Geometry check sheet. Reference: the model listing, model coordinates, mm. A direction names the side the tool comes from. Coordinates: 2 decimals unless noted, no trailing zeros. Loops run counter-clockwise (first coordinate to the right, second up) from the corner with the lowest first, then second, coordinate; pieces in that order, holes last. Notation, with made-up numbers: (-2.5, 11.25) - (48.5, 11.25) arc R29 ccw to (48.5, 46.25) - close; hole circle Ø6 at (81, 89.5). An arc over 180 degrees is marked (long way). Write each question's results on one line, items separated by ' | '. Start each with the question number.
(1) Sectioned sample at B-B (z = -4). Enter the section's corners in (x, y), plus the area to 3 significant figures.
(2) Material ranges on probe 1 along Z at (x, y) = (-8, -0.7); probe 2 along Y at (x, z) = (-9, -3.5); probe 3 along Z at (x, y) = (9, 24), recorded low to high.
(3) Sectioned sample at C-C (y = 19.5). Enter the section's corners in (x, z).
(4) Access from +Z, -Z, +X, -X, +Y, -Y to the whole of each face (thin tool, end or side, straight path). Record for faces 4 (the face through (-9.352, -0.74, 9.474)), 5 (the face through (-4, 0, -4)).
(5) Go/stop test with flat-tipped pins: pin 1 Ø1.8 at (x, y) = (8.5, 16.75) entering from -Z; pin 2 Ø12 at (x, y) = (-7.5, 7.5) entering from -Z; pin 3 Ø13 at (x, z) = (0, 0) entering from +Y. Record where each tip stops, or that it passes through.
(6) Sectioned sample at D-D (x = -8.5). Enter the section's corners in (y, z).
(7) Sectioned sample at A-A (z = 8). Enter the section's corners in (x, y).
(8) Mould release check, pull along X, two halves, no side actions. Record for faces 1 (the face through (-0.309, 33.497, 16.497)), 2 (the face through (9.352, -0.74, -9.474)), 3 (the face through (4, 14, 15.737)): pulls with the +X half, pulls with the -X half, needs draft (parallel to the pull), parting line crosses it, or undercut.
from build123d import *

# Parameters (mm, degrees)
SKETCH1_W                = 30
SKETCH1_H                = 30
SKETCH1_R                = 5
SKETCH1_R_2              = 2
BASE_FLANGE1_DEPTH       = 1.5
EDGE_FLANGE1_DEPTH       = 30
EDGE_FLANGE1_START       = -1.5
EDGE_FLANGE1_PROFILE_R   = 1.5
EDGE_FLANGE1_PROFILE_R_2 = 3.6
EDGE_FLANGE1_FLAT_DEPTH  = 1.5


# Sheet-metal steps are written as plain solids
with BuildPart() as part:
    # Sketch1 → Base-Flange1 (new body)
    with BuildSketch(Plane(origin=(0, 0, 0), x_dir=(1, 0, 0), z_dir=(0, 1, 0))):
        Rectangle(SKETCH1_W, SKETCH1_H)
        with Locations(Location((0, 0, 0), (0, 0, 270))):
            Circle(SKETCH1_R, mode=Mode.SUBTRACT)
        with Locations(Location((8, 8, 0), (0, 0, 270))):
            Circle(SKETCH1_R_2, mode=Mode.SUBTRACT)
        with Locations(Location((8, -8, 0), (0, 0, 270))):
            Circle(SKETCH1_R_2, mode=Mode.SUBTRACT)
        with Locations(Location((-8, -8, 0), (0, 0, 90))):
            Circle(SKETCH1_R_2, mode=Mode.SUBTRACT)
        with Locations(Location((-8, 8, 0), (0, 0, 90))):
            Circle(SKETCH1_R_2, mode=Mode.SUBTRACT)
    extrude(amount=-BASE_FLANGE1_DEPTH)

    # Edge-Flange1 bend section (across the edge) → Edge-Flange1 (add)
    with BuildSketch(Plane(origin=(-15, 0, 15.7366), x_dir=(0, 0, -1), z_dir=(1, 0, 0))):
        with BuildLine():
            Line((-1.5, 0.7366), (0, 0.7366))
            ThreePointArc((0, 0.7366), (0.215745145, 0.215745145), (0.7366, 0))
            Line((0.7366, 0), (0.7366, -1.5))
            ThreePointArc((0.7366, -1.5), (-0.844915027, -0.844915027), (-1.5, 0.7366))
        make_face()
    extrude(amount=EDGE_FLANGE1_DEPTH)

    # Edge-Flange1 profile (on flange) → Edge-Flange1 flat (add)
    with BuildSketch(Plane(origin=(0, 0, 15.7366), x_dir=(-1, 0, 0), z_dir=(0, 0, -1)).offset(EDGE_FLANGE1_START)):
        with BuildLine():
            ThreePointArc((15, 20.067164179), (0, 33.5), (-15, 20.067164179))
            Line((-15, 20.067164179), (-15, 0.7366))
            Line((-15, 0.7366), (15, 0.7366))
            Line((15, 0.7366), (15, 20.067164179))
        make_face()
        with Locations((8.5, 16.75)):
            Circle(EDGE_FLANGE1_PROFILE_R, mode=Mode.SUBTRACT)
        with Locations((0, 16.75)):
            Circle(EDGE_FLANGE1_PROFILE_R_2, mode=Mode.SUBTRACT)
        with Locations((-8.5, 16.75)):
            Circle(EDGE_FLANGE1_PROFILE_R, mode=Mode.SUBTRACT)
    extrude(amount=EDGE_FLANGE1_FLAT_DEPTH)


solid = part.part
Outcome:
1) outline: (-15, -1.5) - (-3, -1.5) - (-3, 0) - (-15, 0) - close; (3, -1.5) - (15, -1.5) - (15, 0) - (3, 0) - close | area: 36.0 mm2
2) probe 1: z = -15 to -10, -6 to 6, 10 to 16.71 | probe 2: y = -1.5 to 0 | probe 3: z = 15.74 to 17.24
3) outline: (-15, 15.74) - (-2.32, 15.74) - (-2.32, 17.24) - (-15, 17.24) - close; (2.32, 15.74) - (15, 15.74) - (15, 17.24) - (2.32, 17.24) - close
4) face 4: +Y, -Y | face 5: -Z, +X, -X, +Y
5) pin 1: passes through | pin 2: stops at z = 15.74 | pin 3: stops at y = 0
6) outline: (-1.5, -15) - (0, -15) - (0, -9.94) - (-1.5, -9.94) - close; (-1.5, -6.06) - (0, -6.06) - (0, 6.06) - (-1.5, 6.06) - close; (-1.5, 9.94) - (0, 9.94) - (0, 15) arc R0.74 cw to (0.74, 15.74) - (15.25, 15.74) - (15.25, 17.24) - (0.74, 17.24) arc R2.24 ccw to (-1.5, 15) - close; (18.25, 15.74) - (30.88, 15.74) - (30.88, 17.24) - (18.25, 17.24) - close
7) outline: (-15, -1.5) - (-10, -1.5) - (-10, 0) - (-15, 0) - close; (-6, -1.5) - (6, -1.5) - (6, 0) - (-6, 0) - close; (10, -1.5) - (15, -1.5) - (15, 0) - (10, 0) - close
8) face 1: parting line crosses it | face 2: undercut | face 3: needs draft
